Work out the finished part from the listing and answer in its coordinate system (mm). Face numbers are marked on the shaded views. A direction names the side the tool comes from. Give positions to 0.01 mm unless a question says otherwise; leave off trailing zeros. Order: outer loops, then holes, each group sorted by start corner. A loop starts at its lowest first (then second) coordinate and runs counter-clockwise, first axis right, second up.
```python
from build123d import *

# Parameters (mm, degrees)
F2_DEPTH = 26.4
F3_DEPTH = 4
F6_D     = 5
F6_DEPTH = 5
F6_TIP   = 1.5021515476
F7_D     = 5
F7_DEPTH = 7
F7_TIP   = 1.5021515476


with BuildPart() as f2:
    # F0 (on Front) → F2 (new body)
    with BuildSketch(Plane.XZ):
        with BuildLine():
            Line((23.6029717884, 8.2401288069), (37.7647548615, 13.1842060911))
            ThreePointArc((37.7647548615, 13.1842060911), (30.9779974122, 25.3054080451), (20.4548362885, 34.3744043208))
            Line((20.4548362885, 34.3744043208), (12.7842726803, 21.4840027005))
            ThreePointArc((12.7842726803, 21.4840027005), (19.3612483826, 15.8158800282), (23.6029717884, 8.2401288069))
        make_face()
    extrude(amount=F2_DEPTH)

    # F1 (on Front) + F0 (on Front) → F3 (join)
    with BuildSketch(Plane.XZ):
        with BuildLine():
            ThreePointArc((11.2501599587, 18.9059223764), (17.0378985767, 13.9179744248), (20.7706151738, 7.2513133501))
            Line((20.7706151738, 7.2513133501), (37.7647548615, 13.1842060911))
            ThreePointArc((37.7647548615, 13.1842060911), (30.9779974122, 25.3054080451), (20.4548362885, 34.3744043208))
            Line((20.4548362885, 34.3744043208), (11.2501599587, 18.9059223764))
        make_face()
    with BuildSketch(Plane.XZ):
        with BuildLine():
            Line((23.6029717884, 8.2401288069), (37.7647548615, 13.1842060911))
            ThreePointArc((37.7647548615, 13.1842060911), (30.9779974122, 25.3054080451), (20.4548362885, 34.3744043208))
            Line((20.4548362885, 34.3744043208), (12.7842726803, 21.4840027005))
            ThreePointArc((12.7842726803, 21.4840027005), (19.3612483826, 15.8158800282), (23.6029717884, 8.2401288069))
        make_face()
    extrude(amount=-F3_DEPTH)

    # F6 (one way)
    with BuildSketch(Plane(origin=(29.109795575, 0, 23.7793052059), x_dir=(0, 1, 0), z_dir=(-0.7744499353, 0, -0.6326352011))):
        with Locations((-5, 0)):
            Circle(F6_D / 2)
    extrude(amount=-F6_DEPTH, mode=Mode.SUBTRACT)
    with Locations(Plane(origin=(29.109795575, 0, 23.7793052059), x_dir=(0, 1, 0), z_dir=(-0.7744499353, 0, -0.6326352011))):
        with Locations((-5, 0)):
            with Locations((0, 0, -(F6_DEPTH + F6_TIP / 2))):  # 118° drill point
                Cone(0, F6_D / 2, F6_TIP, mode=Mode.SUBTRACT)

    # F7
    with Locations(Plane(origin=(29.109795575, 0, 23.7793052059), x_dir=(0, 1, 0), z_dir=(0.7744499353, 0, 0.6326352011))):
        with Locations((-5, 0)):
            Hole(F7_D / 2, depth=F7_DEPTH)
            with Locations((0, 0, -(F7_DEPTH + F7_TIP / 2))):  # 118° drill point
                Cone(0, F7_D / 2, F7_TIP, mode=Mode.SUBTRACT)


solid = f2.part
```
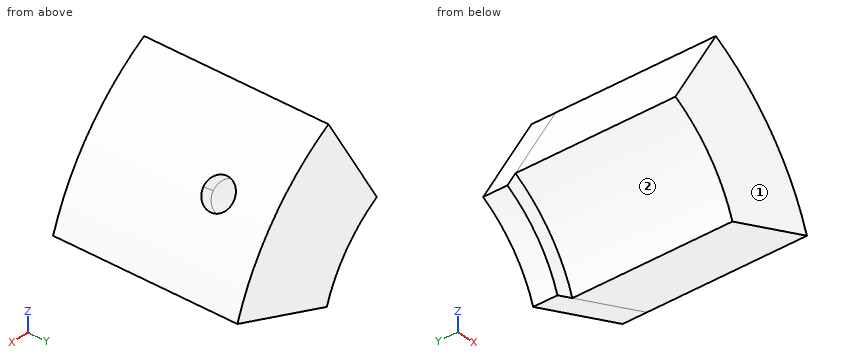
1. The part is cut by section B-B (x = 21.5). Write down the section's boundary in (y, z), then the cut area to 3 significant figures.
Findings below:
outline: (-26.4, 12.76) - (0, 12.76) - (0, 7.51) - (4, 7.51) - (4, 33.73) - (-26.4, 33.73) - close
area: 659 mm2
2. Given P1, Ø6, axis at y = -10.5, z = 17, coming from the -X side; P2, Ø2, axis at x = 33, y = -2.5, coming from the +Z side; P3, Ø5, axis at y = -17.5, z = 30, coming from the -X side, each flat-ended and moving along its own axis, determine where each tip first touches the part or whether it passes through.
Findings below:
P1: stops at x = 15
P2: stops at z = 24
P3: stops at x = 16.36
3. The part is cut by section D-D (x = 33.75). Write down the section's boundary in (y, z), then the cut area to 3 significant figures.
Findings below:
outline: (-26.4, 11.78) - (4, 11.78) - (4, 21.47) - (-26.4, 21.47) - close
area: 294 mm2
4. Straight lines are drawn through the part: probe 1 along Y at (x, z) = (18.25, 17); probe 2 along Z at (x, y) = (24, -4); probe 3 along X at (y, z) = (-6.5, 25). For each, find the intervals that lie inside material, in ascending order.
Findings below:
probe 1: y = 0 to 4
probe 2: z = 8.38 to 18.07, 22.56 to 32
probe 3: x = 14.88 to 27.44
5. The part is cut by section A-A (z = 10.5). Write down the section's boundary in (x, y), then the cut area to 3 significant figures.
Findings below:
outline: (19.33, 0) - (22.69, 0) - (22.69, -26.4) - (30.08, -26.4) - (30.08, 4) - (19.33, 4) - close
area: 238 mm2
6. Which of the six approach directions +Z, -Z, +X, -X, +Y, -Y give full straight-line access (tool end or side, diameter ignored) to the marked faces 1 and 2?
Findings below:
face 1: +Z, -Z, +X, -X, -Y
face 2: -Z, -X, -Y
7. The part is cut by section C-C (y = -10). Write down the section's boundary in (x, z).
Findings below:
outline: (12.78, 21.48) arc R25 cw to (23.6, 8.24) - (37.76, 13.18) arc R40 ccw to (20.45, 34.37) - close
